```python
from build123d import *

# Parameters (mm, degrees)
BOSS_EXTRUDE1_DEPTH                           = 1.25
CSK_FOR_4_FLAT_HEAD_MACHINE_SCREW1_AT_2_COUNT = 2
CSK_FOR_4_FLAT_HEAD_MACHINE_SCREW1_AT_2_PITCH = 65.735474806
CSK_FOR_4_FLAT_HEAD_MACHINE_SCREW1_AT_3_COUNT = 2
CSK_FOR_4_FLAT_HEAD_MACHINE_SCREW1_AT_3_PITCH = 46.482
CSK_FOR_4_FLAT_HEAD_MACHINE_SCREW1_AT_4_COUNT = 2
CSK_FOR_4_FLAT_HEAD_MACHINE_SCREW1_AT_4_PITCH = 46.482
SKETCH7_R                                     = 12.8016
CUT_EXTRUDE1_DEPTH                            = 3.5


with BuildPart() as part:
    # Sketch1 → Boss-Extrude1 (new body, symmetric)
    with BuildSketch(Plane.XY):
        with BuildLine():
            Line((-23.876, 26.797), (23.876, 26.797))
            ThreePointArc((23.876, 26.797), (25.941458908, 25.941458908), (26.797, 23.876))
            Line((26.797, 23.876), (26.797, -23.876))
            ThreePointArc((26.797, -23.876), (25.941458908, -25.941458908), (23.876, -26.797))
            Line((23.876, -26.797), (-23.876, -26.797))
            ThreePointArc((-23.876, -26.797), (-25.941458908, -25.941458908), (-26.797, -23.876))
            Line((-26.797, -23.876), (-26.797, 23.876))
            ThreePointArc((-26.797, 23.876), (-25.941458908, 25.941458908), (-23.876, 26.797))
        make_face()
    extrude(amount=BOSS_EXTRUDE1_DEPTH, both=True)

    # Sketch5 → CSK for #4 Flat Head Machine Screw1 (revolve, cut)
    with BuildSketch(Plane(origin=(-23.241, 23.241, 1.25), x_dir=(0, -1, 0), z_dir=(1, 0, 0))):
        Polygon((0, 0), (0, 2.5), (1.6002, 2.5), (1.6002, 1.957696955), (3.302, 0), align=None)
    csk_for_4_flat_head_machine_screw1 = revolve(axis=Axis((-23.241, 23.241, 7.6), (0, 0, -1)), mode=Mode.SUBTRACT)

    # CSK for #4 Flat Head Machine Screw1 at 2: CSK for #4 Flat Head Machine Screw1 ×2
    with Locations(*[Vector(0.707106781, -0.707106781, 0) * (i * CSK_FOR_4_FLAT_HEAD_MACHINE_SCREW1_AT_2_PITCH) for i in range(1, CSK_FOR_4_FLAT_HEAD_MACHINE_SCREW1_AT_2_COUNT)]):
        add(csk_for_4_flat_head_machine_screw1, mode=Mode.SUBTRACT)

    # CSK for #4 Flat Head Machine Screw1 at 3: CSK for #4 Flat Head Machine Screw1 ×2
    with Locations(*[(i * CSK_FOR_4_FLAT_HEAD_MACHINE_SCREW1_AT_3_PITCH, 0, 0) for i in range(1, CSK_FOR_4_FLAT_HEAD_MACHINE_SCREW1_AT_3_COUNT)]):
        add(csk_for_4_flat_head_machine_screw1, mode=Mode.SUBTRACT)

    # CSK for #4 Flat Head Machine Screw1 at 4: CSK for #4 Flat Head Machine Screw1 ×2
    with Locations(*[(0, -i * CSK_FOR_4_FLAT_HEAD_MACHINE_SCREW1_AT_4_PITCH, 0) for i in range(1, CSK_FOR_4_FLAT_HEAD_MACHINE_SCREW1_AT_4_COUNT)]):
        add(csk_for_4_flat_head_machine_screw1, mode=Mode.SUBTRACT)

    # Sketch7 → Cut-Extrude1 (cut, through all)
    with BuildSketch(Plane.XY.offset(1.25)):
        with Locations((0, 5.08)):
            Circle(SKETCH7_R)
    extrude(amount=-CUT_EXTRUDE1_DEPTH, mode=Mode.SUBTRACT)


solid = part.part
```
For this review, take the finished solid that the model builds, in its own axes (mm). Coordinates: 2 decimals unless noted, no trailing zeros. Write each loop counter-clockwise with the first axis right and the second up, starting at its lowest first coordinate (ties: lowest second). Pieces come first, ordered by that corner, then holes.
(1) Wall thickness on probe 1 along X at (y, z) = (-21.5, -0.35); probe 2 along Y at (x, z) = (-23.5, -0.35); probe 3 along X at (y, z) = (-24, 1.15): over which ranges is each line inside the solid? List them lowest first.
(2) Add section C-C on z = 0.7. Give the boundary of the cut face in (x, y).
(3) The part is to be moulded in two halves that separate along X. For faces 1 (the face through (21.802, 22.324, -0.585)), 2 (the face through (-21.821, 22.503, -0.975)), 3 (the face through (0, 26.797, 0)), 4 (the face through (25.92, 25.96, 0.02)), say which applies: +X half, -X half, draft (parallel to the pull), parting line (faces both ways), or undercut.
(4) For pin 1 Ø4 at (x, y) = (-23.241, 23.241) entering from +Z; pin 2 Ø3.5 at (x, y) = (23.241, -23.241) entering from +Z, all flat-tipped, find the tip position at first contact; note any pin that passes through.
(5) Add section B-B on x = 0. Give the boundary of the cut face in (y, z), then the cut area to 3 significant figures.
(6) Add section A-A on y = 5.08. Give the boundary of the cut face in (x, z), then the cut area to 3 significant figures.
Answer sheet:
1. probe 1: x = -26.8 to -24.03, -22.45 to 22.45, 24.03 to 26.8
1. probe 2: y = -26.8 to -25.13, -21.35 to 21.35, 25.13 to 26.8
1. probe 3: x = -26.79 to -26.37, -20.12 to 20.12, 26.37 to 26.79
2. outline: (-26.8, -23.88) arc R2.92 ccw to (-23.88, -26.8) - (23.88, -26.8) arc R2.92 ccw to (26.8, -23.88) - (26.8, 23.88) arc R2.92 ccw to (23.88, 26.8) - (-23.88, 26.8) arc R2.92 ccw to (-26.8, 23.88) - close; hole circle Ø5.65 at (-23.24, -23.24); hole circle Ø5.65 at (-23.24, 23.24); hole circle Ø25.6 at (0, 5.08); hole circle Ø5.65 at (23.24, -23.24); hole circle Ø5.65 at (23.24, 23.24)
3. face 1: undercut
3. face 2: undercut
3. face 3: draft
3. face 4: +X half
4. pin 1: stops at z = -0.25
4. pin 2: stops at z = -0.54
5. outline: (-26.8, -1.25) - (-7.72, -1.25) - (-7.72, 1.25) - (-26.8, 1.25) - close; (17.88, -1.25) - (26.8, -1.25) - (26.8, 1.25) - (17.88, 1.25) - close
5. area: 70.0 mm2
6. outline: (-26.8, -1.25) - (-12.8, -1.25) - (-12.8, 1.25) - (-26.8, 1.25) - close; (12.8, -1.25) - (26.8, -1.25) - (26.8, 1.25) - (12.8, 1.25) - close
6. area: 70.0 mm2
